```python
from build123d import *

# Parameters (mm, degrees)
SKETCH1_R           = 11
SKETCH1_R_2         = 4
BOSS_EXTRUDE1_DEPTH = 2
SKETCH2_R           = 1.5
CUT_EXTRUDE1_DEPTH  = 2
SKETCH3_R           = 5.5
SKETCH3_R_2         = 4
BOSS_EXTRUDE2_DEPTH = 10


with BuildPart() as part:
    # Sketch1 → Boss-Extrude1 (new body)
    with BuildSketch(Plane(origin=(0, 0, 0), x_dir=(1, 0, 0), z_dir=(0, 1, 0))):
        with Locations(Location((0, 0, 0), (0, 0, 270))):
            Circle(SKETCH1_R)
        with Locations(Location((0, 0, 0), (0, 0, 270))):
            Circle(SKETCH1_R_2, mode=Mode.SUBTRACT)
    extrude(amount=BOSS_EXTRUDE1_DEPTH)

    # Sketch2 → Cut-Extrude1 (cut)
    with BuildSketch(Plane(origin=(0, 2, 0), x_dir=(1, 0, 0), z_dir=(0, 1, 0))):
        with Locations(Location((8, 0, 0), (0, 0, 270))):
            Circle(SKETCH2_R)
        with Locations(Location((-8, 0, 0), (0, 0, 270))):
            Circle(SKETCH2_R)
        with Locations(Location((0, 8, 0), (0, 0, 270))):
            Circle(SKETCH2_R)
        with Locations(Location((0, -8, 0), (0, 0, 270))):
            Circle(SKETCH2_R)
    extrude(amount=-CUT_EXTRUDE1_DEPTH, mode=Mode.SUBTRACT)

    # Sketch3 → Boss-Extrude2 (add)
    with BuildSketch(Plane(origin=(0, 2, 0), x_dir=(1, 0, 0), z_dir=(0, 1, 0))):
        with Locations(Location((0, 0, 0), (0, 0, 270))):
            Circle(SKETCH3_R)
        with Locations(Location((0, 0, 0), (0, 0, 270))):
            Circle(SKETCH3_R_2, mode=Mode.SUBTRACT)
    extrude(amount=BOSS_EXTRUDE2_DEPTH)


solid = part.part
```
Could you check a few things on this model? Use its own coordinates, in mm. A direction names the side the tool comes from. Round coordinates to 2 decimals unless told otherwise and drop trailing zeros. Order: outer loops, then holes, each group sorted by start corner. A loop starts at its lowest first (then second) coordinate and runs counter-clockwise, first axis right, second up. Notation, with made-up numbers: (-40, 20) -> (-23, 20) arc R25 ccw to (-23, 33) -> close; hole circle Ø2 at (49, 89). An arc over 180 degrees is marked (long way). One line per question, with ' | ' between items.
Q1. Which directions (+Z, -Z, +X, -X, +Y, -Y) give clear straight access to the entire face, cutting with the end or side of a thin tool? Please do faces 4 (the face through (-5.37, 6.93, -1.19)), 5 (the face through (0.07, 1.01, -9.5)).
Computed values:
face 4: +Y | face 5: +Y, -Y
Q2. I'm going to push flat-ended pins straight in: pin 1 (6 mm diameter, centred on x = -6.5, z = 6.5, fed in from +Y); pin 2 (2 mm diameter, centred on y = 4.5, z = -5, fed in from -X); pin 3 (1.5 mm diameter, centred on y = 3.5, z = -4.5, fed in from +X). Where does each tip first touch, or does it pass through?
Computed values:
pin 1: y = 2 | pin 2: x = -3.77 | pin 3: x = 4.02
Q3. If we section it at C-C on y = 1.5: Write out the boundary of the cut face in (x, z).
Computed values:
outline: circle Ø22 at (0, 0); hole circle Ø3 at (-8, 0); hole circle Ø8 at (0, 0); hole circle Ø3 at (0, -8); hole circle Ø3 at (0, 8); hole circle Ø3 at (8, 0)
Q4. If I drill on line 1 (X direction, y = 1.05, z = 0); line 2 (Y direction, x = 9, z = -2.5); line 3 (Z direction, x = 3, y = 7), over which ranges is the centre line in solid material (lowest first)? Write a range as from..to.
Computed values:
line 1: -11..-9.5, -6.5..-4, 4..6.5, 9.5..11 | line 2: 0..2 | line 3: -4.61..-2.65, 2.65..4.61
Q5. If we section it at B-B on x = 0: Write out the boundary of the cut face in (y, z).
Computed values:
outline: (0, -11) -> (2, -11) -> (2, -9.5) -> (0, -9.5) -> close; (0, -6.5) -> (2, -6.5) -> (2, -5.5) -> (12, -5.5) -> (12, -4) -> (0, -4) -> close; (0, 4) -> (12, 4) -> (12, 5.5) -> (2, 5.5) -> (2, 6.5) -> (0, 6.5) -> close; (0, 9.5) -> (2, 9.5) -> (2, 11) -> (0, 11) -> close
Q6. We'd pull the mould along Z, two halves only. Please class faces 1 (the face through (-10.74, 0.99, -2.38)), 2 (the face through (0.07, 1.01, 6.5)), 3 (the face through (-2, 12, -4)): released by +Z, released by -Z, zero draft, split by the parting line, or undercut.
Computed values:
face 1: split by the parting line | face 2: undercut | face 3: zero draft
Q7. If we section it at D-D on z = -8: Write out the boundary of the cut face in (x, y).
Computed values:
outline: (-7.55, 0) -> (-1.5, 0) -> (-1.5, 2) -> (-7.55, 2) -> close; (1.5, 0) -> (7.55, 0) -> (7.55, 2) -> (1.5, 2) -> close
Q8. If we section it at A-A on z = 0: Write out the boundary of the cut face in (x, y).
Computed values:
outline: (-11, 0) -> (-9.5, 0) -> (-9.5, 2) -> (-11, 2) -> close; (-6.5, 0) -> (-4, 0) -> (-4, 12) -> (-5.5, 12) -> (-5.5, 2) -> (-6.5, 2) -> close; (4, 0) -> (6.5, 0) -> (6.5, 2) -> (5.5, 2) -> (5.5, 12) -> (4, 12) -> close; (9.5, 0) -> (11, 0) -> (11, 2) -> (9.5, 2) -> close
